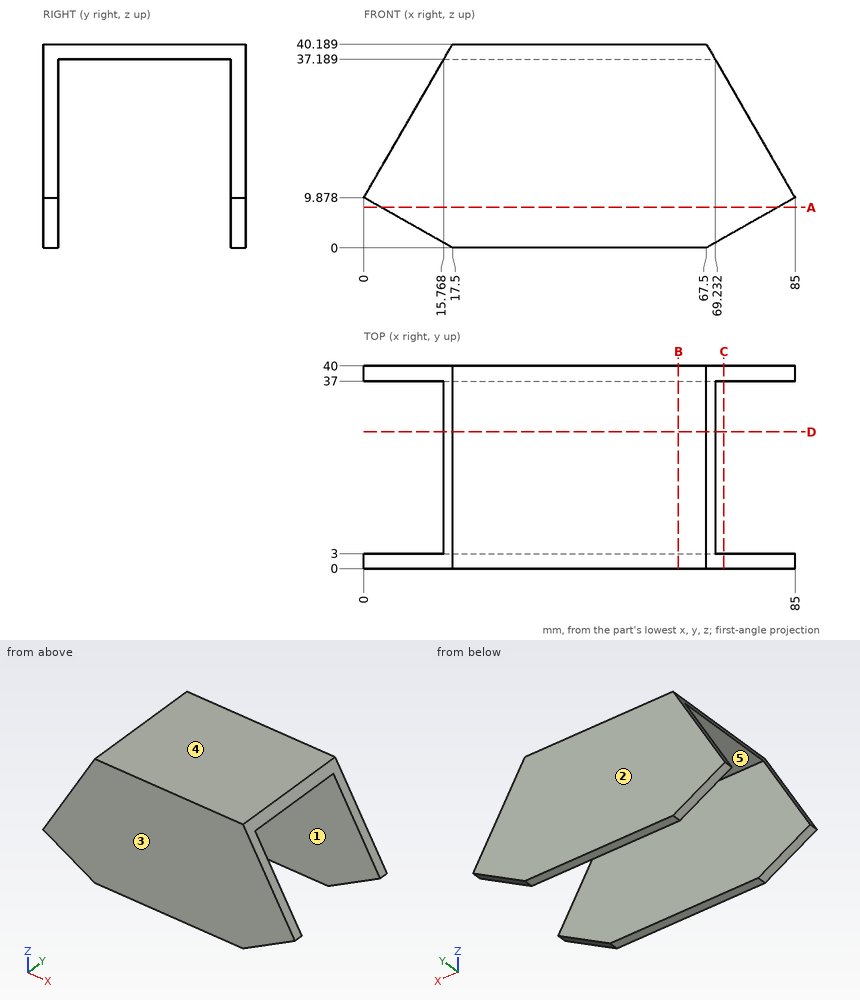
Job drawing, mm, ordinate dimensions from the low corner. One solid piece. A direction names the side the tool comes from. Give positions to 0.01 mm unless a question says otherwise; leave off trailing zeros. Loops run counter-clockwise (first coordinate to the right, second up) from the corner with the lowest first, then second, coordinate; pieces in that order, holes last. Notation, with made-up numbers: (20.25, 60.5) -> (72.25, 60.5) arc R26 ccw to (72.25, 79.5) -> close; hole circle Ø10 at (88, 69.25). An arc over 180 degrees is marked (long way). Write each question's results on one line, items separated by ' | '.
(1) Cut at D-D on y = 27. List the corners of the cut face in (x, z), and give its area (3 significant figures).
Geometry results:
outline: (15.77, 37.19) -> (69.23, 37.19) -> (67.5, 40.19) -> (17.5, 40.19) -> close | area: 155 mm²
(2) Probe line 1 along Y through (x, z) = (56, 30); line 2 along Z through (x, y) = (42, 19.5); line 3 along Z through (x, y) = (16, 25.5). List the from-to ranges inside material, lowest first.
Geometry results:
line 1: y = 0 to 3, 37 to 40 | line 2: z = 37.19 to 40.19 | line 3: z = 37.19 to 37.59
(3) Tool access for the marked faces 1 and 2: list every direction of +Z, -Z, +X, -X, +Y, -Y with a clear straight run to the whole face (end or side of a thin tool).
Geometry results:
face 1: -Z, +X, -X | face 2: +Z, -Z, +X, -X, +Y
(4) Cut at B-B on x = 62. List the corners of the cut face in (y, z), and give its area (3 significant figures).
Geometry results:
outline: (0, 0) -> (3, 0) -> (3, 37.19) -> (37, 37.19) -> (37, 0) -> (40, 0) -> (40, 40.19) -> (0, 40.19) -> close | area: 343 mm²
(5) Pull direction Y, two halves, no side cores. Call the marked faces 3, 4 and 5: released by +Y, released by -Y, zero draft, split by the parting line, or undercut.
Geometry results:
face 3: released by -Y | face 4: zero draft | face 5: undercut
(6) Cut at C-C on x = 71. List the corners of the cut face in (y, z) (1 decimal).
Geometry results:
outline: (0, 2) -> (3, 2) -> (3, 34.1) -> (0, 34.1) -> close; (37, 2) -> (40, 2) -> (40, 34.1) -> (37, 34.1) -> close
(7) Flat gauge pin, fed straight in: pin 1 Ø3 at (x, y) = (39.5, 20) entering from -Z. Where does the tip first touch, or does it go through?
Geometry results:
pin 1: stops at z = 37.19
(8) Cut at A-A on z = 8. List the corners of the cut face in (x, y), and give its area (3 significant figures).
Geometry results:
outline: (3.33, 0) -> (81.67, 0) -> (81.67, 3) -> (3.33, 3) -> close; (3.33, 37) -> (81.67, 37) -> (81.67, 40) -> (3.33, 40) -> close | area: 470 mm²
